from build123d import *

# Parameters (mm, degrees)
ESQUISSE1_R             = 30.75
BOSS_EXTRU_1_DEPTH      = 8
ESQUISSE2_R             = 3
BOSS_EXTRU_2_DEPTH      = 56
ESQUISSE4_R             = 30.75
BOSS_EXTRU_4_DEPTH      = 4.5
ESQUISSE6_R             = 3
BOSS_EXTRU_5_DEPTH      = 40
ESQUISSE12_R            = 4
ENL_V_MAT_EXTRU_1_DEPTH = 6
ENL_V_START             = -10
ENL_V_MAT_EXTRU_2_DEPTH = 10
ESQUISSE15_R            = 10
ENL_V_MAT_EXTRU_3_DEPTH = 10
ESQUISSE18_R            = 30.75
BOSS_EXTRU_10_DEPTH     = 4.5
ESQUISSE19_R            = 2.05
ENL_V_MAT_EXTRU_4_DEPTH = 62
ESQUISSE20_R            = 3.5
ENL_V_MAT_EXTRU_5_DEPTH = 10


with BuildPart() as part:
    # Esquisse1 → Boss.-Extru.1 (new body)
    with BuildSketch(Plane.XY):
        Circle(ESQUISSE1_R)
    extrude(amount=BOSS_EXTRU_1_DEPTH)

    # Esquisse2 → Boss.-Extru.2 (add)
    with BuildSketch(Plane.XY.offset(8)):
        with Locations((0, 27.5)):
            Circle(ESQUISSE2_R)
        with Locations((27.5, 0)):
            Circle(ESQUISSE2_R)
        with Locations((-27.5, 0)):
            Circle(ESQUISSE2_R)
        with Locations((0, -27.5)):
            Circle(ESQUISSE2_R)
    extrude(amount=BOSS_EXTRU_2_DEPTH)

    # Esquisse4 → Boss.-Extru.4 (add)
    with BuildSketch(Plane.XY.offset(64)):
        Circle(ESQUISSE4_R)
    extrude(amount=BOSS_EXTRU_4_DEPTH)

    # Esquisse6 → Boss.-Extru.5 (add)
    with BuildSketch(Plane.XY.offset(68.5)):
        with Locations((0, -27.5)):
            Circle(ESQUISSE6_R)
        with Locations((-27.5, 0)):
            Circle(ESQUISSE6_R)
        with Locations((0, 27.5)):
            Circle(ESQUISSE6_R)
        with Locations((27.5, 0)):
            Circle(ESQUISSE6_R)
    extrude(amount=BOSS_EXTRU_5_DEPTH)

    # Esquisse12 → Enlèv. mat.-Extru.1 (cut)
    with BuildSketch(Plane.XY.offset(68.5)):
        with Locations((9.98690327, 23.224420757)):
            Circle(ESQUISSE12_R)
    extrude(amount=-ENL_V_MAT_EXTRU_1_DEPTH, mode=Mode.SUBTRACT)

    # Esquisse13 → Enlèv. mat.-Extru.2 (cut)
    with BuildSketch(Plane.XY.offset(68.5).offset(ENL_V_START)):
        with BuildLine():
            Line((-15.652440464, 26.468162149), (-15.269059678, 25.645999401))
            ThreePointArc((-15.269059678, 25.645999401), (-7.818437842, 16.76669406), (-9.831212956, 28.181708971))
            Line((-9.831212956, 28.181708971), (-10.214593742, 29.003871719))
            ThreePointArc((-10.214593742, 29.003871719), (-12.995511549, 27.868964451), (-15.652440464, 26.468162149))
        make_face()
    extrude(amount=ENL_V_MAT_EXTRU_2_DEPTH, mode=Mode.SUBTRACT)

    # Esquisse15 → Enlèv. mat.-Extru.3 (cut)
    with BuildSketch(Plane.XY.offset(68.5)):
        Circle(ESQUISSE15_R)
    extrude(amount=-ENL_V_MAT_EXTRU_3_DEPTH, mode=Mode.SUBTRACT)

    # Esquisse18 → Boss.-Extru.10 (add)
    with BuildSketch(Plane.XY.offset(108.5)):
        Circle(ESQUISSE18_R)
    extrude(amount=BOSS_EXTRU_10_DEPTH)

    # Esquisse19 → Enlèv. mat.-Extru.4 (cut)
    with BuildSketch(Plane.ZY.offset(30.75)):
        with Locations((4, 0.25)):
            Circle(ESQUISSE19_R)
    extrude(amount=-ENL_V_MAT_EXTRU_4_DEPTH, mode=Mode.SUBTRACT)

    # Esquisse20 → Enlèv. mat.-Extru.5 (cut)
    with BuildSketch(Plane.XY.offset(113)):
        with Locations((21.297953152, 14.912987345)):
            Circle(ESQUISSE20_R)
        with Locations((-14.912987345, 21.297953152)):
            Circle(ESQUISSE20_R)
        with Locations((-21.297953152, -14.912987345)):
            Circle(ESQUISSE20_R)
        with Locations((14.912987345, -21.297953152)):
            Circle(ESQUISSE20_R)
    extrude(amount=-ENL_V_MAT_EXTRU_5_DEPTH, mode=Mode.SUBTRACT)


solid = part.part
Build history of the part. All positions in model axes, mm. A direction names the side the tool comes from. Round coordinates to 2 decimals unless told otherwise and drop trailing zeros. Write each loop counter-clockwise with the first axis right and the second up, starting at its lowest first coordinate (ties: lowest second). Pieces come first, ordered by that corner, then holes. Notation, with made-up numbers: (-22.5, 59) - (35.5, 59) arc R15 ccw to (35.5, 86) - close; hole circle Ø4 at (-32.5, 23). An arc over 180 degrees is marked (long way). Use CSV: the item, a comma, the result in double quotes.
(1) Band-saw the part on C-C (z = 46). Write the cut outline in (x, y), plus the area to 3 significant figures.
Response:
outline,"circle Ø6 at (-27.5, 0); circle Ø6 at (0, -27.5); circle Ø6 at (0, 27.5); circle Ø6 at (27.5, 0)"
area,"113 mm²"
(2) Pin check, flat tips, straight feed: P1, Ø8, axis at y = 19.5, z = 28.5, coming from the +X side; P2, Ø10, axis at y = 21, z = 43, coming from the +X side. Stop position of each tip, or through.
Response:
P1,"through"
P2,"x = 2.6"
(3) Wall check: line 1 (Z direction, x = 6.5, y = 0.25); line 2 (Z direction, x = -16, y = -8.5); line 3 (Z direction, x = -17.5, y = 20). Give the ranges that are in metal, low to high.
Response:
line 1,"0 to 1.95, 6.05 to 8, 108.5 to 113"
line 2,"0 to 8, 64 to 68.5, 108.5 to 113"
line 3,"0 to 8, 64 to 68.5"
(4) Band-saw the part on A-A (x = -20). Write the cut outline in (y, z).
Response:
outline,"(-23.36, 0) - (23.36, 0) - (23.36, 8) - (-23.36, 8) - close; (-23.36, 64) - (23.36, 64) - (23.36, 68.5) - (-23.36, 68.5) - close; (-23.36, 108.5) - (-18.16, 108.5) - (-18.16, 113) - (-23.36, 113) - close; (-11.66, 108.5) - (23.36, 108.5) - (23.36, 113) - (-11.66, 113) - close; hole circle Ø4.1 at (0.25, 4)"
(5) Band-saw the part on D-D (y = -27.5). Write the cut outline in (x, z).
Response:
outline,"(-13.76, 0) - (13.76, 0) - (13.76, 8) - (3, 8) - (3, 64) - (13.76, 64) - (13.76, 68.5) - (3, 68.5) - (3, 108.5) - (13.76, 108.5) - (13.76, 113) - (-13.76, 113) - (-13.76, 108.5) - (-3, 108.5) - (-3, 68.5) - (-13.76, 68.5) - (-13.76, 64) - (-3, 64) - (-3, 8) - (-13.76, 8) - close"
(6) 3-axis set-ups, long thin cutter, end or side, ignore diameter. For faces 4 (the flat face through (0, 0, 0)), 5 (the flat face through (0, -13, 64)), 6 (the cylindrical face through (14.154, -24.715, 110.782)): which of +Z, -Z, +X, -X, +Y, -Y reach the whole face in a straight line?
Response:
face 4,"-Z, +X, -X, +Y, -Y"
face 5,"none"
face 6,"+Z"
(7) Mould opens along Y. For faces 1 (the cylindrical face through (18.52, 12.783, 110.782)), 2 (the flat face through (0, 0, 113)), 3 (the cylindrical face through (11.796, -28.397, 66.218)) say: pulls with the +Y half, pulls with the -Y half, needs draft (parallel to the pull), parting line crosses it, or undercut.
Response:
face 1,"undercut"
face 2,"needs draft"
face 3,"parting line crosses it"
(8) Band-saw the part on B-B (x = 0). Give the number of separate pieces and of enclosed holes in the cut face, plus the area to 3 significant figures.
Response:
separate pieces,"1"
enclosed holes,"2"
area,"2,090 mm²"
